Geometry: final body of the model. Coordinates: model frame, mm. Give positions to 0.01 mm unless a question says otherwise; leave off trailing zeros. Write each loop counter-clockwise with the first axis right and the second up, starting at its lowest first coordinate (ties: lowest second). Pieces come first, ordered by that corner, then holes. Notation, with made-up numbers: (-24.75, -5.5) -> (14.25, -5.5) arc R20 ccw to (14.25, 11.5) -> close; hole circle Ø3 at (79, 53). An arc over 180 degrees is marked (long way). Answer in a Markdown table with one row per item. Add a question column.
Item 1: First-contact query: P1, Ø4.5, axis at x = 277, y = -3, coming from the +Z side. Flat tip, straight axial feed; report the tip coordinate or a pass-through.
Item 2: Section query A-A on x = -163.5. Output: boundary loops of the cut face in (y, z), plus the area to 3 significant figures.
Item 3: Material intervals for probe 1 along Y at (x, z) = (219.5, 0.4); probe 2 along Y at (x, z) = (114, 2.3); probe 3 along Y at (x, z) = (335, 2.6), sorted ascending. Write a range as from..to.
Item 4: Section query B-B on z = 2.45. State how many separate pieces and enclosed holes the cut face has, plus the area to 3 significant figures.
```python
from build123d import *

# Parameters (mm, degrees)
SKETCH_1_R          = 3.25
EXTRUDE_1_DEPTH     = 4
HOLE_WIZARD_M32_D   = 3.4
HOLE_WIZARD_M52_D   = 5.5
HOLE_WIZARD_M53_D   = 5.5
FILLET_5_R          = 10
CUT_EXTRUDE_4_DEPTH = 354.032576401
FILLET_7_R          = 6
HOLE_WIZARD_M34_D   = 3.4
CUT_EXTRUDE_5_DEPTH = 354.032576401


with BuildPart() as part:
    # Эскиз1 → Бобышка-Вытянуть1 (new body)
    with BuildSketch(Plane.XY):
        with BuildLine():
            Line((-349.818316726, 28.672449915), (-342.910885265, -15.303620822))
            Line((-342.910885265, -15.303620822), (-240, -46))
            Line((-240, -46), (240, -46))
            Line((240, -46), (342.910885265, -15.303620822))
            Line((342.910885265, -15.303620822), (349.818316726, 28.672449915))
            ThreePointArc((349.818316726, 28.672449915), (346.399852001, 40.749019149), (335, 46))
            Line((335, 46), (-335, 46))
            ThreePointArc((-335, 46), (-346.399852001, 40.749019149), (-349.818316726, 28.672449915))
        make_face()
        with Locations((-335, -9.635315981)):
            Circle(SKETCH_1_R, mode=Mode.SUBTRACT)
        with Locations(Location((335, -9.635315981, 0), (0, 0, 180))):
            Circle(SKETCH_1_R, mode=Mode.SUBTRACT)
    extrude(amount=EXTRUDE_1_DEPTH)

    # Отверстие с зазором M32 (through all)
    with Locations(Plane.XY.offset(4)):
        with Locations((-335, 41), (-345, 31), (-335, 21), (-325, 31), (325, 31), (335, 41), (345, 31), (335, 21)):
            Hole(HOLE_WIZARD_M32_D / 2)

    # Отверстие с зазором M52 (through all)
    with Locations(Plane(origin=(0, 0, 0), x_dir=(-1, 0, 0), z_dir=(0, 0, -1))):
        with Locations((215, -7)):
            Hole(HOLE_WIZARD_M52_D / 2)

    # Отверстие с зазором M53 (through all)
    with Locations(Plane(origin=(0, 0, 0), x_dir=(-1, 0, 0), z_dir=(0, 0, -1))):
        with Locations((31.771314746, 9.83), (35.189476411, 32.040691677), (33.141482074, 20.990703059), (31.085819286, -1.380913569), (31.085819286, -12.619086431), (31.771893326, -23.836297834), (33.141482074, -34.990703059)):
            Hole(HOLE_WIZARD_M53_D / 2)

    # Скругление5
    fillet_5_edges = [part.edges().sort_by_distance(p)[0] for p in [
        (342.910885265, -15.303620822, 2),
        (240, -46, 2),
        (-240, -46, 2),
        (-342.910885265, -15.303620822, 2),
    ]]
    fillet(fillet_5_edges, radius=FILLET_5_R)

    # Эскиз22 → Вырез-Вытянуть4 (cut, through all)
    with BuildSketch(Plane(origin=(0, 0, 0), x_dir=(-1, 0, 0), z_dir=(0, 0, -1))):
        Polygon((-227.540368898, -36), (-98.70593747, -36), (-79.540368898, -30.283271798), (-79.540368898, 36), (-208.374800326, 36), (-227.540368898, 30.283271798), align=None)
        with BuildLine():
            Line((227.54, -30.283271798), (208.374431428, -36))
            Line((208.374431428, -36), (40.898736363, -36))
            ThreePointArc((40.898736363, -36), (38.644905491, 0.150569256), (43.818079226, 36))
            Line((43.818079226, 36), (227.54, 36))
            Line((227.54, 36), (227.54, -30.283271798))
        make_face()
        Polygon((-271, 30.283271798), (-251.834431428, 36), (-239.540368898, 36), (-239.540368898, -35.701718831), (-271, -26.317903284), align=None)
        Polygon((-67.540368898, -36), (-13.70593747, -36), (5.459631102, -30.283271798), (5.459631102, 36), (-48.374800326, 36), (-67.540368898, 30.283271798), align=None)
        Polygon((239.54, 30.283271798), (258.705568572, 36), (271, 36), (271, -26.317903284), (239.54, -35.701828866), align=None)
    extrude(amount=-CUT_EXTRUDE_4_DEPTH, mode=Mode.SUBTRACT)

    # Скругление7
    fillet_7_edges = [part.edges().sort_by_distance(p)[0] for p in [
        (227.540368898, -36, 2),
        (227.540368898, 30.283271798, 2),
        (208.374800326, 36, 2),
        (79.540368898, 36, 2),
        (79.540368898, -30.283271798, 2),
        (98.70593747, -36, 2),
        (271, -26.317903284, 2),
        (271, 30.283271798, 2),
        (251.834431428, 36, 2),
        (239.540368898, 36, 2),
        (239.540368898, -35.701718831, 2),
        (-40.898736363, -36, 2),
        (-43.818079226, 36, 2),
        (-227.54, 36, 2),
        (-227.54, -30.283271798, 2),
        (-208.374431428, -36, 2),
        (67.540368898, -36, 2),
        (67.540368898, 30.283271798, 2),
        (48.374800326, 36, 2),
        (-5.459631102, 36, 2),
        (-5.459631102, -30.283271798, 2),
        (13.70593747, -36, 2),
        (-271, -26.317903284, 2),
        (-239.54, -35.701828866, 2),
        (-239.54, 30.283271798, 2),
        (-258.705568572, 36, 2),
        (-271, 36, 2),
    ]]
    fillet(fillet_7_edges, radius=FILLET_7_R)

    # Отверстие с зазором M34 (through all)
    with Locations(Plane(origin=(0, 0, 0), x_dir=(-1, 0, 0), z_dir=(0, 0, -1))):
        with Locations((-233.540368898, 32), (-233.540368898, -28), (-73.540368898, -28), (-73.540368898, 32), (11.459631102, 32), (11.459631102, -28), (277, 32), (277, -3), (-277, 32), (-277, -3), (233.54, -28), (233.54, 32)):
            Hole(HOLE_WIZARD_M34_D / 2)

    # Эскиз25 → Вырез-Вытянуть5 (cut, through all)
    with BuildSketch(Plane.XY.offset(4)):
        with BuildLine():
            Line((-208.641482074, -37.3), (-203.641482074, -37.3))
            ThreePointArc((-203.641482074, -37.3), (-201.941482074, -39), (-203.641482074, -40.7))
            Line((-203.641482074, -40.7), (-208.641482074, -40.7))
            ThreePointArc((-208.641482074, -40.7), (-210.341482074, -39), (-208.641482074, -37.3))
        make_face()
        with BuildLine():
            Line((-177.141482074, -37.3), (-172.141482074, -37.3))
            ThreePointArc((-172.141482074, -37.3), (-170.441482074, -39), (-172.141482074, -40.7))
            Line((-172.141482074, -40.7), (-177.141482074, -40.7))
            ThreePointArc((-177.141482074, -40.7), (-178.841482074, -39), (-177.141482074, -37.3))
        make_face()
        with BuildLine():
            Line((-140.641482074, -40.7), (-145.641482074, -40.7))
            ThreePointArc((-145.641482074, -40.7), (-147.341482074, -39), (-145.641482074, -37.3))
            Line((-145.641482074, -37.3), (-140.641482074, -37.3))
            ThreePointArc((-140.641482074, -37.3), (-138.941482074, -39), (-140.641482074, -40.7))
        make_face()
    extrude(amount=-CUT_EXTRUDE_5_DEPTH, mode=Mode.SUBTRACT)


solid = part.part
```
Findings below:
| question | item | result |
|---|---|---|
| 1 | P1 | stops at z = 4 |
| 2 | outline | (-46, 0) -> (-36, 0) -> (-36, 4) -> (-46, 4) -> close; (36, 0) -> (46, 0) -> (46, 4) -> (36, 4) -> close |
| 2 | area | 80.0 mm^2 |
| 3 | probe 1 | y = -46..-36, 32.68..46 |
| 3 | probe 2 | y = -46..-36, 36..46 |
| 3 | probe 3 | y = -17.66..-12.89, -6.39..19.3, 22.7..39.3, 42.7..46 |
| 4 | separate pieces | 1 |
| 4 | enclosed holes | 37 |
| 4 | area | 26,800 mm^2 |
